Verification items for the finished model (mm, model axes). A direction names the side the tool comes from. Round coordinates to 2 decimals unless told otherwise and drop trailing zeros. Order: outer loops, then holes, each group sorted by start corner. A loop starts at its lowest first (then second) coordinate and runs counter-clockwise, first axis right, second up. Notation, with made-up numbers: M 36,-26.5 L 64,-26.5 A15 ccw 64,-10.5 Z; hole C 61.25,45 d8. An arc over 180 degrees is marked long. Answer as a JSON object with one key per item and string values. Group by question number.
```python
from build123d import *

# Parameters (mm, degrees)
F0_W     = 95.25
F0_H     = 180.975
F1_DEPTH = 11.43
F2_W     = 76.2
F2_H     = 127
F2_W_2   = 60.96
F2_H_2   = 111.76
F2_H_3   = 25.4
F2_H_4   = 10.16
F3_DEPTH = 11.303
F4_R     = 5.08


with BuildPart() as f1:
    # F0 (on Top) → F1 (new body)
    with BuildSketch(Plane.XY):
        with Locations((47.625, 90.4875)):
            Rectangle(F0_W, F0_H)
    extrude(amount=F1_DEPTH)

    # F2 (on face) → F3 (cut)
    with BuildSketch(Plane.XY.offset(11.43)):
        with Locations((47.625, 107.95)):
            Rectangle(F2_W, F2_H)
        with Locations((47.625, 107.95)):
            Rectangle(F2_W_2, F2_H_2, mode=Mode.SUBTRACT)
        with Locations((47.625, 22.225)):
            Rectangle(F2_W, F2_H_3)
        with Locations((47.625, 22.225)):
            Rectangle(F2_W_2, F2_H_4, mode=Mode.SUBTRACT)
    extrude(amount=-F3_DEPTH, mode=Mode.SUBTRACT)

    # F4
    f4_edges = [f1.edges().sort_by_distance(p)[0] for p in [
        (0, 0, 5.715),
        (9.525, 34.925, 5.7785),
        (95.25, 0, 5.715),
        (85.725, 34.925, 5.7785),
        (9.525, 9.525, 5.7785),
        (85.725, 9.525, 5.7785),
        (85.725, 44.45, 5.7785),
        (9.525, 44.45, 5.7785),
        (0, 180.975, 5.715),
        (95.25, 180.975, 5.715),
        (85.725, 171.45, 5.7785),
        (9.525, 171.45, 5.7785),
    ]]
    fillet(f4_edges, radius=F4_R)


solid = f1.part
```
Q1. Cross-section at A-A, the plane z = 8.75. Give the number of separate pieces and of enclosed holes in the cut face, then the cut area to 3 significant figures.
Q2. Thickness scan on line 1 (Y direction, x = 49, z = 3.5) (3 decimals); line 2 (X direction, y = 54.5, z = 4.75) (3 decimals); line 3 (X direction, y = 50.5, z = 3) (3 decimals). Record the ranges inside material, lowest first. Write a range as from..to.
Q3. Release check for a two-part mould opening along Y. For faces 1 (the face through (93.722, 1.449, 5.795)), 2 (the face through (47, 109, 11.43)), 3 (the face through (78.105, 107, 6)) record: released by +Y, released by -Y, zero draft, split by the parting line, or undercut.
Q4. Tool access check on faces 4 (the face through (47, 0, 6)), 5 (the face through (84.2, 45.9, 5.7)). Record the directions out of +Z, -Z, +X, -X, +Y, -Y that give a thin tool (end or side, any length) a straight path to the whole face; none if there is none.
Q5. Cross-section at B-B, the plane y = 104. Record the cut outline in (x, z) (3 decimals), then the cut area to 3 significant figures.
Q6. Cross-section at C-C, the plane x = 76. Record the cut outline in (y, z) (3 decimals).
Conclusion:
{
 "1": {"separate pieces": "3", "enclosed holes": "2", "area": "13,100 mm2"},
 "2": {"line 1": "0..9.525, 17.145..27.305, 34.925..44.45, 52.07..163.83, 171.45..180.975", "line 2": "0..9.525, 17.145..78.105, 85.725..95.25", "line 3": "0..9.525, 85.725..95.25"},
 "3": {"face 1": "released by -Y", "face 2": "zero draft", "face 3": "undercut"},
 "4": {"face 4": "+Z, -Z, +X, -X, -Y", "face 5": "+Z"},
 "5": {"outline": "M 0,0 L 95.25,0 L 95.25,11.43 L 85.725,11.43 L 85.725,0.127 L 78.105,0.127 L 78.105,11.43 L 17.145,11.43 L 17.145,0.127 L 9.525,0.127 L 9.525,11.43 L 0,11.43 Z", "area": "916 mm2"},
 "6": {"outline": "M 0,0 L 180.975,0 L 180.975,11.43 L 171.45,11.43 L 171.45,0.127 L 163.83,0.127 L 163.83,11.43 L 52.07,11.43 L 52.07,0.127 L 44.45,0.127 L 44.45,11.43 L 34.925,11.43 L 34.925,0.127 L 27.305,0.127 L 27.305,11.43 L 17.145,11.43 L 17.145,0.127 L 9.525,0.127 L 9.525,11.43 L 0,11.43 Z"}
}
